from build123d import *

# Parameters (mm, degrees)
SKETCH_1_W          = 180
SKETCH_1_H          = 115
EXTRUDE_1_DEPTH     = 3
CUT_EXTRUDE_3_REACH = 108.842
SKETCH_7_W          = 76.2
SKETCH_7_H          = 20.5
SKETCH_8_W          = 81.2
SKETCH_8_H          = 25.5
SKETCH_8_W_2        = 76.2
SKETCH_8_H_2        = 20.5
EXTRUDE_2_DEPTH     = 25
SKETCH_9_W          = 81.2
SKETCH_9_H          = 25.5
EXTRUDE_3_DEPTH     = 2.5
CUT_EXTRUDE_START   = -3
SKETCH_4_W          = 4
SKETCH_4_H          = 8
CUT_EXTRUDE_2_DEPTH = 1.6


with BuildPart() as part:
    # 草图1 → 凸台-拉伸1 (new body)
    with BuildSketch(Plane.XY):
        Rectangle(SKETCH_1_W, SKETCH_1_H)
    extrude(amount=EXTRUDE_1_DEPTH)

    # 草图7 → 电池位切除-拉伸3 (cut, up to next)
    with BuildSketch(Plane(origin=(0, 0, 0), x_dir=(-1, 0, 0), z_dir=(0, 0, -1)), mode=Mode.PRIVATE) as cut_extrude_3_sk1:
        with Locations((30, 40.25)):
            Rectangle(SKETCH_7_W, SKETCH_7_H)
    cut_extrude_3_tool1 = extrude(cut_extrude_3_sk1.sketch, amount=-CUT_EXTRUDE_3_REACH, mode=Mode.PRIVATE) & part.part
    cut_extrude_3 = cut_extrude_3_tool1.solids().sort_by_distance((-30, 40.25, 0))[0]
    add(cut_extrude_3, mode=Mode.SUBTRACT)

    # 草图8 → 凸台-拉伸2 (add)
    with BuildSketch(Plane.XY.offset(3)):
        with Locations((-30, 40.25)):
            Rectangle(SKETCH_8_W, SKETCH_8_H)
        with Locations((-30, 40.25)):
            Rectangle(SKETCH_8_W_2, SKETCH_8_H_2, mode=Mode.SUBTRACT)
    extrude_2 = extrude(amount=EXTRUDE_2_DEPTH)

    # 草图9 → 凸台-拉伸3 (add)
    with BuildSketch(Plane.XY.offset(28)):
        with Locations((-30, 40.25)):
            Rectangle(SKETCH_9_W, SKETCH_9_H)
    extrude_3 = extrude(amount=-EXTRUDE_3_DEPTH)

    # 草图4 → 切除-拉伸2 (cut)
    with BuildSketch(Plane(origin=(0, 0, 0), x_dir=(-1, 0, 0), z_dir=(0, 0, -1)).offset(CUT_EXTRUDE_START)):
        with Locations((70.1, 40.25)):
            Rectangle(SKETCH_4_W, SKETCH_4_H)
    cut_extrude_2 = extrude(amount=CUT_EXTRUDE_2_DEPTH, mode=Mode.SUBTRACT)

    # 镜向1: 电池位切除-拉伸3, 凸台-拉伸2, 凸台-拉伸3, 切除-拉伸2 across plane
    add(cut_extrude_3.mirror(Plane.ZX), mode=Mode.SUBTRACT)
    add(extrude_2.mirror(Plane.ZX))
    add(extrude_3.mirror(Plane.ZX))
    add(cut_extrude_2.mirror(Plane.ZX), mode=Mode.SUBTRACT)


solid = part.part
Design review of the part built by this model. Coordinates are the model's own, in mm. A direction names the side the tool comes from. Coordinates: 2 decimals unless noted, no trailing zeros. Write each loop counter-clockwise with the first axis right and the second up, starting at its lowest first coordinate (ties: lowest second). Pieces come first, ordered by that corner, then holes. Notation, with made-up numbers: (23.5, 70) -> (37.5, 70) arc R27 ccw to (37.5, 94) -> close; hole circle Ø4 at (-4.5, 45). An arc over 180 degrees is marked (long way). Write each question's results on one line, items separated by ' | '. Start each with the question number.
(1) Tool access review of faces 1 (the face through (-70.6, 40, 15)), 2 (the face through (-31, 27.5, 15)), 3 (the face through (10.6, -40, 15)), 4 (the face through (-70, -40, 1.4)), 5 (the face through (-31, 40, 25.5)): name each direction out of +Z, -Z, +X, -X, +Y, -Y from which nothing blocks a thin tool from reaching the whole face with its end or side.
(2) The part is to be moulded in two halves that separate along X. For faces 6 (the face through (10.6, 40, 15)), 7 (the face through (-1, 1, 0)), 8 (the face through (-68.1, -40, 13)), 9 (the face through (-70.6, -40, 15)), say which applies: pulls with the +X half, pulls with the -X half, needs draft (parallel to the pull), parting line crosses it, or undercut.
(3) For line 1 along Y through (x, z) = (-54.5, 7.25); line 2 along X through (y, z) = (42, 7.5); line 3 along Z through (x, y) = (22, -18.5), list the stretches that pass through material, from the lowest coordinate up. Write a range as from..to.
(4) Take a section at A-A on z = 5.25. Write out the cut boundary in (x, y), and give its area (3 significant figures).
(5) Clearance check with flat-ended pins moving along their axes: P1, Ø1.5, axis at x = -49, z = 4.5, coming from the -Y side; P2, Ø16.5, axis at y = -38.5, z = 14, coming from the -X side; P3, Ø0.8, axis at x = -69, y = 40.5, coming from the -Z side; P4, Ø7.5, axis at x = -39, z = 10, coming from the +Y side. State where each tip first meets the part, or that it passes through.
(6) Take a section at D-D on x = 34. Write out the cut boundary in (y, z), and give its area (3 significant figures).
(7) Take a section at B-B on y = 46. Write out the cut boundary in (x, z).
(8) Take a section at C-C on x = -53. Write out the cut boundary in (y, z), and give its area (4 significant figures).
Results found:
1) face 1: +Z, -X, +Y, -Y | face 2: +Z, +X, -X | face 3: +Z, +X, +Y, -Y | face 4: none | face 5: -Z
2) face 6: pulls with the +X half | face 7: needs draft | face 8: undercut | face 9: pulls with the -X half
3) line 1: y = -53..-50.5, -30..-27.5, 27.5..30, 50.5..53 | line 2: x = -70.6..-68.1, 8.1..10.6 | line 3: z = 0..3
4) outline: (-70.6, -53) -> (10.6, -53) -> (10.6, -27.5) -> (-70.6, -27.5) -> close; (-70.6, 27.5) -> (10.6, 27.5) -> (10.6, 53) -> (-70.6, 53) -> close; hole (-68.1, -50.5) -> (8.1, -50.5) -> (8.1, -30) -> (-68.1, -30) -> close; hole (-68.1, 30) -> (8.1, 30) -> (8.1, 50.5) -> (-68.1, 50.5) -> close | area: 1,020 mm2
5) P1: stops at y = -53 | P2: stops at x = -70.6 | P3: stops at z = 0 | P4: stops at y = 53
6) outline: (-57.5, 0) -> (57.5, 0) -> (57.5, 3) -> (-57.5, 3) -> close | area: 345 mm2
7) outline: (-90, 0) -> (-68.1, 0) -> (-68.1, 25.5) -> (8.1, 25.5) -> (8.1, 0) -> (90, 0) -> (90, 3) -> (10.6, 3) -> (10.6, 28) -> (-70.6, 28) -> (-70.6, 3) -> (-90, 3) -> close
8) outline: (-57.5, 0) -> (-50.5, 0) -> (-50.5, 25.5) -> (-30, 25.5) -> (-30, 0) -> (30, 0) -> (30, 25.5) -> (50.5, 25.5) -> (50.5, 0) -> (57.5, 0) -> (57.5, 3) -> (53, 3) -> (53, 28) -> (27.5, 28) -> (27.5, 3) -> (-27.5, 3) -> (-27.5, 28) -> (-53, 28) -> (-53, 3) -> (-57.5, 3) -> close | area: 574.5 mm2
